```python
from build123d import *

# Parameters (mm, degrees)
SKETCH1_R               = 1.5
BOSS_EXTRUDE1_DEPTH     = 21
SKETCH2_R               = 2
BOSS_EXTRUDE2_DEPTH     = 123
FILLET1_R               = 5
FILLET2_R               = 0.5
CUT_EXTRUDE1_DEPTH      = 129.195163715
CUT_EXTRUDE1_DEPTH_BACK = 129.195163715
SKETCH4_R               = 0.75
SKETCH4_R_2             = 1
CUT_EXTRUDE2_DEPTH      = 129.195163715
CUT_EXTRUDE2_DEPTH_BACK = 129.195163715
SKETCH5_R               = 1


with BuildPart() as part:
    # Sketch1 → Boss-Extrude1 (new body)
    with BuildSketch(Plane.XY):
        with Locations(Location((0, 0, 0), (0, 0, 180))):
            Circle(SKETCH1_R)
    extrude(amount=BOSS_EXTRUDE1_DEPTH)

    # Sketch2 → Boss-Extrude2 (add)
    with BuildSketch(Plane(origin=(0, 0, 0), x_dir=(-1, 0, 0), z_dir=(0, 0, -1))):
        Circle(SKETCH2_R)
    extrude(amount=BOSS_EXTRUDE2_DEPTH)

    # Sketch3 → Revolve1 (revolve)
    with BuildSketch(Plane(origin=(0, 0, 0), x_dir=(1, 0, 0), z_dir=(0, 1, 0))):
        with BuildLine():
            Line((-5, 123), (5, 123))
            ThreePointArc((5, 123), (0, 128), (-5, 123))
        make_face()
    revolve(axis=Axis((-5, 0, -123), (1, 0, 0)))

    # Fillet1
    fillet1_edges = [part.edges().sort_by_distance(p)[0] for p in [
        (2, 0, -118.417424305),
    ]]
    fillet(fillet1_edges, radius=FILLET1_R)

    # Fillet2
    fillet2_edges = [part.edges().sort_by_distance(p)[0] for p in [
        (1.5, 0, 21),
    ]]
    fillet(fillet2_edges, radius=FILLET2_R)

    # Sketch4 → Cut-Extrude1 (cut, two sides: drawn at the far end of the back side and taken through both)
    with BuildSketch(Plane(origin=(0, 0, 0), x_dir=(1, 0, 0), z_dir=(0, 1, 0)).offset(-CUT_EXTRUDE1_DEPTH_BACK)):
        with Locations(Location((0, -15.5, 0), (0, 0, 270))):
            Circle(SKETCH4_R)
        with Locations(Location((0, 34.5, 0), (0, 0, 270))):
            Circle(SKETCH4_R_2)
        with Locations(Location((0, 113.5, 0), (0, 0, 270))):
            Circle(SKETCH4_R_2)
    extrude(amount=CUT_EXTRUDE1_DEPTH + CUT_EXTRUDE1_DEPTH_BACK, mode=Mode.SUBTRACT)

    # Sketch5 → Cut-Extrude2 (cut, two sides: drawn at the far end of the back side and taken through both)
    with BuildSketch(Plane(origin=(0, 0, 0), x_dir=(0, 0, -1), z_dir=(1, 0, 0)).offset(-CUT_EXTRUDE2_DEPTH_BACK)):
        with Locations((3, 0)):
            Circle(SKETCH5_R)
    extrude(amount=CUT_EXTRUDE2_DEPTH + CUT_EXTRUDE2_DEPTH_BACK, mode=Mode.SUBTRACT)


solid = part.part
```
Here's how the part is built. I have some questions about the finished solid (model axes, mm). Give positions to 0.01 mm unless a question says otherwise; leave off trailing zeros. Loops run counter-clockwise (first coordinate to the right, second up) from the corner with the lowest first, then second, coordinate; pieces in that order, holes last. Notation, with made-up numbers: M -37.5,-21.5 L 19.5,-21.5 A18 cw 19.5,-11.5 Z; hole C 40,89 d1. An arc over 180 degrees is marked long. Put each result on its own line as item: value. Start each with the question number.
(1) Will these pins go through, and if not, where does the flat tip stop? pin 1 Ø1 at (x, y) = (2.5, -3.5) entering from -Z; pin 2 Ø5 at (y, z) = (-2, -20.5) entering from +X; pin 3 Ø2 at (x, y) = (-2.5, -2) entering from -Z; pin 4 Ø3 at (x, y) = (-1, 1) entering from +Z.
(2) I want a section at B-B on z = -104. Please give me the cut outline in (x, y), then the cut area to 3 significant figures.
(3) I want a section at A-A on z = 9. Please give me the cut outline in (x, y).
(4) I need wall thicknesses on line 1 along Y through (x, z) = (-0.1, -3); line 2 along Z through (x, y) = (0, -1.05); line 3 along Z through (x, y) = (0, 0.8). Which ranges of each line are inside material? Lowest first, please. Write a range as [from, to].
Answer block:
1. pin 1: z = -126.25
1. pin 2: x = 2
1. pin 3: z = -127.49
1. pin 4: z = 21
2. outline: C 0,0 d4
2. area: 12.6 mm^2
3. outline: C 0,0 d3
4. line 1: [-2, -1], [1, 2]
4. line 2: [-127.89, -114.5], [-112.5, -35.5], [-33.5, 14.75], [16.25, 21]
4. line 3: [-127.94, -114.5], [-112.5, -35.5], [-33.5, -3.6], [-2.4, 14.75], [16.25, 21]
